```python
from build123d import *

# Parameters (mm, degrees)
F0_W     = 8
F0_H     = 8
F1_DEPTH = 2.5
F3_DEPTH = 3.5
F4_SIZE  = 0.75
F5_R     = 0.5


with BuildPart() as f1:
    # F0 (on Top) → F1 (new body)
    with BuildSketch(Plane.XY):
        with Locations((4, 4)):
            Rectangle(F0_W, F0_H)
    extrude(amount=F1_DEPTH)

    # F2 (on face) → F3 (join)
    with BuildSketch(Plane.XY.offset(2.5)):
        with BuildLine():
            Line((2.460592, 3.167699), (4.832301, 5.539408))
            ThreePointArc((4.832301, 5.539408), (2.762563, 5.237437), (2.460592, 3.167699))
        make_face()
        with BuildLine():
            ThreePointArc((3.167699, 2.460592), (4.896095, 2.496832), (5.75, 4))
            ThreePointArc((5.75, 4), (5.696535, 4.429265), (5.539408, 4.832301))
            Line((5.539408, 4.832301), (3.167699, 2.460592))
        make_face()
    extrude(amount=F3_DEPTH)

    # F4
    f4_edges = [f1.edges().sort_by_distance(p)[0] for p in [
        (5.237437, 2.762563, 6),
        (2.762563, 5.237437, 6),
    ]]
    chamfer(f4_edges, length=F4_SIZE)

    # F5
    f5_edges = [f1.edges().sort_by_distance(p)[0] for p in [
        (0, 4, 2.5),
        (4, 0, 2.5),
        (8, 4, 2.5),
        (4, 8, 2.5),
        (4, 8, 0),
        (8, 4, 0),
        (4, 0, 0),
        (0, 4, 0),
    ]]
    fillet(f5_edges, radius=F5_R)


solid = f1.part
```
CAD build for the part. Positions are in the model's coordinates, mm. A direction names the side the tool comes from. Round coordinates to 2 decimals unless told otherwise and drop trailing zeros. Order: outer loops, then holes, each group sorted by start corner. A loop starts at its lowest first (then second) coordinate and runs counter-clockwise, first axis right, second up. Notation, with made-up numbers: (-27, 8.5) - (-4, 8.5) arc R28 cw to (-4, 47.5) - close; hole circle Ø4 at (-11.75, 52). An arc over 180 degrees is marked (long way). Answer in a Markdown table with one row per item. Add a question column.
(1) Band-saw the part on A-A on y = 6.75. List the corners of the cut face in (x, z).
(2) Probe L1, parallel to Y at x = 3.5, z = 2.05; L2, parallel to Z at x = 4.75, y = 1.75; L3, parallel to Y at x = 3.5, z = 2.75. List the from-to ranges inside material, lowest first. Write a range as [from, to].
(3) Band-saw the part on B-B on z = 3.15. List the corners of the cut face in (x, y).
(4) 3-axis set-ups, long thin cutter, end or side, ignore diameter. For faces 5 (the face through (4, 4, 2.5)), 6 (the face through (5.7, 4.42, 3.86)), 7 (the face through (4.9, 2.5, 3.9)), 8 (the face through (8, 4, 1)): which of +Z, -Z, +X, -X, +Y, -Y reach the whole face in a straight line?
(5) Band-saw the part on D-D on z = 5.65. List the corners of the cut face in (x, y), and give its area (3 significant figures).
(6) Mould opens along Y. For faces 1 (the face through (3.5, 4.5, 6)), 2 (the face through (4, 0, 1)), 3 (the face through (3.63, 4.337, 4.226)), 4 (the face through (3.165, 4.866, 5.797)) say: +Y half, -Y half, draft (parallel to the pull), parting line (faces both ways), or undercut.
(7) Drop flat-ended pins along their axis: pin 1 Ø1.5 at (y, z) = (2, 3.5) entering from +X; pin 2 Ø1.5 at (y, z) = (6, 4) entering from -X. Give the stop position or say it passes through.
Data:
| question | item | result |
|---|---|---|
| 1 | outline | (0, 0.5) arc R0.5 ccw to (0.5, 0) - (7.5, 0) arc R0.5 ccw to (8, 0.5) - (8, 2) arc R0.5 ccw to (7.5, 2.5) - (0.5, 2.5) arc R0.5 ccw to (0, 2) - close |
| 2 | L1 | y = [0, 8] |
| 2 | L2 | z = [0, 2.5] |
| 2 | L3 | y = [2.32, 2.79], [4.21, 5.68] |
| 3 | outline | (2.46, 3.17) - (4.83, 5.54) arc R1.75 ccw to start; (3.17, 2.46) arc R1.75 ccw to (5.75, 4) arc R1.75 ccw to (5.54, 4.83) - close |
| 4 | face 5 | +Z |
| 4 | face 6 | +Z, +X, +Y |
| 4 | face 7 | +Z, -Y |
| 4 | face 8 | +Z, -Z, +X, +Y, -Y |
| 5 | outline | (2.76, 3.47) - (4.53, 5.24) arc R1.35 ccw to start; (3.47, 2.76) arc R1.35 ccw to (5.35, 4) arc R1.35 ccw to (5.24, 4.53) - close |
| 5 | area | 3.09 mm^2 |
| 6 | face 1 | draft |
| 6 | face 2 | -Y half |
| 6 | face 3 | undercut |
| 6 | face 4 | parting line |
| 7 | pin 1 | stops at x = 5.22 |
| 7 | pin 2 | stops at x = 2.78 |
